Here's how the part is built. I have some questions about the finished solid (model axes, mm). Face numbers are marked on the shaded views. A direction names the side the tool comes from. Round coordinates to 2 decimals unless told otherwise and drop trailing zeros. Loops run counter-clockwise (first coordinate to the right, second up) from the corner with the lowest first, then second, coordinate; pieces in that order, holes last. Notation, with made-up numbers: M -32.5,14.5 L 3.5,14.5 A30 ccw 3.5,44.5 Z; hole C -37,77 d7. An arc over 180 degrees is marked long. Answer as CSV lines item,"result".
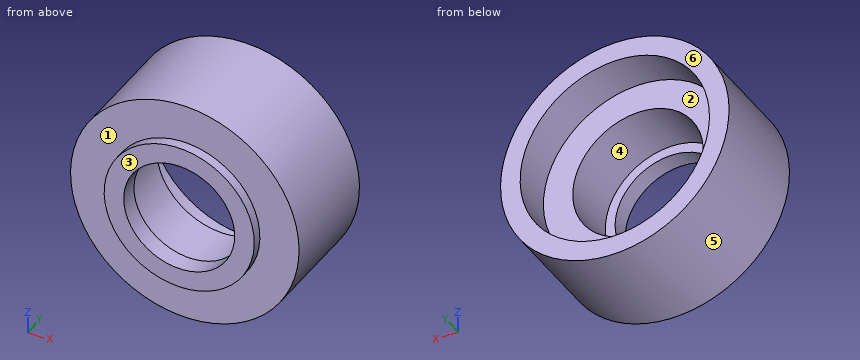
```python
from build123d import *

# Parameters (mm, degrees)
ESQUISSE3_R               = 3.5
SHAPE_DEPTH               = 3.75
ESQUISSE4_R               = 2.9
CUT_EXTRUDE_5_4D_DEPTH    = 3
ESQUISSE5_R               = 1.7
CUT_EXTRUDE_3D_DEPTH      = 3
ESQUISSE6_R               = 3.5
ESQUISSE6_R_2             = 2.3
ENL_V_MAT_EXTRU_2_DEPTH   = 0.5
BOSS_EXTRU_1_START        = 1.75
ESQUISSE9_R               = 2.9
ESQUISSE9_R_2             = 2
BOSS_EXTRU_1_DEPTH        = 1.75
ESQUISSE10_R              = 2.619168903
ERRORPRINTERREMOVER_DEPTH = 0.2


with BuildPart() as part:
    # Esquisse3 → Shape (new body)
    with BuildSketch(Plane(origin=(0, 0, 0), x_dir=(1, 0, 0), z_dir=(0, 1, 0))):
        with Locations(Location((0, 0, 0), (0, 0, 270))):
            Circle(ESQUISSE3_R)
    extrude(amount=SHAPE_DEPTH)

    # Esquisse4 → 5_4D (cut)
    with BuildSketch(Plane(origin=(0, 3.75, 0), x_dir=(1, 0, 0), z_dir=(0, 1, 0))):
        with Locations(Location((0, 0, 0), (0, 0, 270))):
            Circle(ESQUISSE4_R)
    extrude(amount=-CUT_EXTRUDE_5_4D_DEPTH, mode=Mode.SUBTRACT)

    # Esquisse5 → 3D (cut)
    with BuildSketch(Plane(origin=(0, 0.75, 0), x_dir=(1, 0, 0), z_dir=(0, 1, 0))):
        with Locations(Location((0, 0, 0), (0, 0, 270))):
            Circle(ESQUISSE5_R)
    extrude(amount=-CUT_EXTRUDE_3D_DEPTH, mode=Mode.SUBTRACT)

    # Esquisse6 → Enlèv. mat.-Extru.2 (cut)
    with BuildSketch(Plane.XZ):
        with Locations(Location((0, 0, 0), (0, 0, 270))):
            Circle(ESQUISSE6_R)
        with Locations(Location((0, 0, 0), (0, 0, 270))):
            Circle(ESQUISSE6_R_2, mode=Mode.SUBTRACT)
    extrude(amount=-ENL_V_MAT_EXTRU_2_DEPTH, mode=Mode.SUBTRACT)

    # Esquisse9 → Boss.-Extru.1 (add)
    with BuildSketch(Plane(origin=(0, 0.75, 0), x_dir=(1, 0, 0), z_dir=(0, 1, 0)).offset(BOSS_EXTRU_1_START)):
        with Locations(Location((0, 0, 0), (0, 0, 270))):
            Circle(ESQUISSE9_R)
        with Locations(Location((0, 0, 0), (0, 0, 270))):
            Circle(ESQUISSE9_R_2, mode=Mode.SUBTRACT)
    extrude(amount=-BOSS_EXTRU_1_DEPTH)

    # Esquisse10 → ErrorPrinterRemover (cut)
    with BuildSketch(Plane.XZ):
        Circle(ESQUISSE10_R)
    extrude(amount=-ERRORPRINTERREMOVER_DEPTH, mode=Mode.SUBTRACT)


solid = part.part
```
1. I want a section at D-D, the plane z = -2.75. Please give me the cut outline in (x, y), and give its area (3 significant figures).
Evaluation:
outline,"M -2.17,0.5 L 2.17,0.5 L 2.17,3.75 L 0.92,3.75 L 0.92,2.5 L -0.92,2.5 L -0.92,3.75 L -2.17,3.75 Z"
area,"11.8 mm²"
2. We'd pull the mould along Z, two halves only. Please class the marked faces 4, 5 and 6: pulls with the +Z half, pulls with the -Z half, needs draft (parallel to the pull), parting line crosses it, or undercut.
Evaluation:
face 4,"undercut"
face 5,"parting line crosses it"
face 6,"needs draft"
3. I want a section at C-C, the plane y = 1.9. Please give me the cut outline in (x, z).
Evaluation:
outline,"C 0,0 d7; hole C 0,0 d4"
4. Which directions (+Z, -Z, +X, -X, +Y, -Y) give clear straight access to the entire face, cutting with the end or side of a thin tool? Please do the marked faces 1, 2 and 3.
Evaluation:
face 1,"-Y"
face 2,"+Y"
face 3,"+Z, -Z, +X, -X, -Y"
5. I want a section at B-B, the plane z = 0. Please give me the cut outline in (x, y).
Evaluation:
outline,"M -3.5,0.5 L -2.3,0.5 L -2.3,0.2 L -1.7,0.2 L -1.7,0.75 L -2,0.75 L -2,2.5 L -2.9,2.5 L -2.9,3.75 L -3.5,3.75 Z; M 1.7,0.2 L 2.3,0.2 L 2.3,0.5 L 3.5,0.5 L 3.5,3.75 L 2.9,3.75 L 2.9,2.5 L 2,2.5 L 2,0.75 L 1.7,0.75 Z"
6. For P1, Ø1.5, axis at x = -1, y = 1, coming from the -Z side; P2, Ø3, axis at x = 0, z = 0, coming from the -Y side; P3, Ø3, axis at x = 0.5, z = 0.5, coming from the +Y side; P4, Ø1, axis at x = 1.5, y = 1, coming from the +Z side, each with a flat end and sliding along its axis, tell me the tip position at first contact or that it passes through.
Evaluation:
P1,"stops at z = -3.49"
P2,"passes through"
P3,"stops at y = 2.5"
P4,"stops at z = 3.35"
7. If I drill on line 1 (X direction, y = 3.4, z = 0); line 2 (X direction, y = 2.1, z = 0); line 3 (Y direction, x = 1.75, z = -0.75), over which ranges is the centre line in solid material (lowest first)? Write a range as [from, to].
Evaluation:
line 1,"x = [-3.5, -2.9], [2.9, 3.5]"
line 2,"x = [-3.5, -2], [2, 3.5]"
line 3,"y = [0.2, 0.75]"
8. I want a section at A-A, the plane x = 0. Please give me the cut outline in (y, z), and give its area (3 significant figures).
Evaluation:
outline,"M 0.2,-2.3 L 0.5,-2.3 L 0.5,-3.5 L 3.75,-3.5 L 3.75,-2.9 L 2.5,-2.9 L 2.5,-2 L 0.75,-2 L 0.75,-1.7 L 0.2,-1.7 Z; M 0.2,1.7 L 0.75,1.7 L 0.75,2 L 2.5,2 L 2.5,2.9 L 3.75,2.9 L 3.75,3.5 L 0.5,3.5 L 0.5,2.3 L 0.2,2.3 Z"
area,"8.01 mm²"
